from build123d import *

# Parameters (mm, degrees)
F2_W     = 23.7
F2_H     = 1.7
F3_DEPTH = 7.5
F4_R     = 2
F5_R     = 2


with BuildPart() as f1:
    # F0 (on Front) → F1 (revolve)
    with BuildSketch(Plane.XZ):
        Polygon((0, -1.5), (0, 0), (-11.85, 0), (-11.85, -6.5), (-16.75, -6.5), (-16.75, -9.2), (-19, -9.2), (-19, -10.7), (-15.25, -10.7), (-15.25, -8), (-10.35, -8), (-10.35, -1.5), align=None)
    revolve(axis=Axis((0, 0, -0.75), (0, 0, 1)))

    # F2 (on Top) → F3 (join)
    with BuildSketch(Plane.XY):
        Rectangle(F2_W, F2_H)
    extrude(amount=F3_DEPTH)

    # F4
    f4_edges = [f1.edges().sort_by_distance(p)[0] for p in [
        (-11.85, 0, 7.5),
    ]]
    fillet(f4_edges, radius=F4_R)

    # F5
    f5_edges = [f1.edges().sort_by_distance(p)[0] for p in [
        (11.85, 0, 7.5),
    ]]
    fillet(f5_edges, radius=F5_R)


solid = f1.part
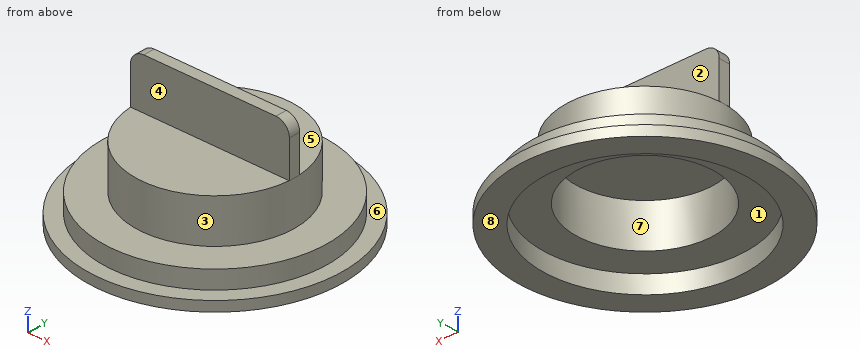
Could you check a few things on this model? Use its own coordinates, in mm. Face numbers are marked on the shaded views. A direction names the side the tool comes from. Give positions to 0.01 mm unless a question says otherwise; leave off trailing zeros. Write each loop counter-clockwise with the first axis right and the second up, starting at its lowest first coordinate (ties: lowest second). Pieces come first, ordered by that corner, then holes. Notation, with made-up numbers: (73, 39) - (126, 39) arc R7 cw to (126, 44) - close; hole circle Ø5 at (-21, 14). An arc over 180 degrees is marked (long way). Use CSV: the item, a comma, the result in double quotes. Start each with the question number.
Item 1: If I drill on line 1 along X through (y, z) = (0, -5.75); line 2 along X through (y, z) = (0, -8.95); line 3 along Y through (x, z) = (0, -9.8), over which ranges is the centre line in solid material (lowest first)?
Item 2: If we mould it in two halves opening along X, with no side actions, what happens to the marked faces 1, 2 and 3? For each: pulls with the +X half, pulls with the -X half, needs draft (parallel to the pull), parting line crosses it, or undercut.
Item 3: For the marked faces 4, 5, 6, 7 and 8, which set-ups out of +Z, -Z, +X, -X, +Y, -Y let a thin tool reach every point of the face, with its end or its side?
Item 4: I want a section at B-B, the plane y = -4.5. Please give me the cut outline in (x, z).
Item 5: I want a section at A-A, the plane x = 0. Please give me the cut outline in (y, z), then the cut area to 4 significant figures.
Item 6: I'm going to push flat-ended pins straight in: pin 1 (3 mm diameter, centred on y = -5.5, z = -6.5, fed in from -X); pin 2 (1.5 mm diameter, centred on x = 6.5, z = -4, fed in from -Y); pin 3 (16.5 mm diameter, centred on x = 0, y = 0, fed in from -Z); pin 4 (10 mm diameter, centred on x = -8, y = -5, fed in from +Z). Where does each tip first touch, or does it pass through?
Item 7: I want a section at C-C, the plane z = -8.5. Please give me the cut outline in (x, y).
Item 8: I want a section at D-D, the plane z = 4.5. Please give me the cut outline in (x, y).
Findings:
1,line 1,"x = -11.85 to -10.35, 10.35 to 11.85"
1,line 2,"x = -16.75 to -15.25, 15.25 to 16.75"
1,line 3,"y = -19 to -15.25, 15.25 to 19"
2,face 1,"undercut"
2,face 2,"needs draft"
2,face 3,"parting line crosses it"
3,face 4,"+Z, +X, -X, -Y"
3,face 5,"+Z, +X, -X, +Y"
3,face 6,"+Z"
3,face 7,"-Z"
3,face 8,"-Z, +X, -X, +Y, -Y"
4,outline,"(-18.46, -10.7) - (-14.57, -10.7) - (-14.57, -8) - (-9.32, -8) - (-9.32, -1.5) - (9.32, -1.5) - (9.32, -8) - (14.57, -8) - (14.57, -10.7) - (18.46, -10.7) - (18.46, -9.2) - (16.13, -9.2) - (16.13, -6.5) - (10.96, -6.5) - (10.96, 0) - (-10.96, 0) - (-10.96, -6.5) - (-16.13, -6.5) - (-16.13, -9.2) - (-18.46, -9.2) - close"
5,outline,"(-19, -10.7) - (-15.25, -10.7) - (-15.25, -8) - (-10.35, -8) - (-10.35, -1.5) - (10.35, -1.5) - (10.35, -8) - (15.25, -8) - (15.25, -10.7) - (19, -10.7) - (19, -9.2) - (16.75, -9.2) - (16.75, -6.5) - (11.85, -6.5) - (11.85, 0) - (0.85, 0) - (0.85, 7.5) - (-0.85, 7.5) - (-0.85, 0) - (-11.85, 0) - (-11.85, -6.5) - (-16.75, -6.5) - (-16.75, -9.2) - (-19, -9.2) - close"
5,area,"97.35 mm2"
6,pin 1,"stops at x = -16.27"
6,pin 2,"stops at y = -10.36"
6,pin 3,"stops at z = -1.5"
6,pin 4,"stops at z = 7.5"
7,outline,"circle Ø33.5 at (0, 0); hole circle Ø30.5 at (0, 0)"
8,outline,"(-11.85, -0.85) - (11.85, -0.85) - (11.85, 0.85) - (-11.85, 0.85) - close"
